from build123d import *

# Parameters (mm, degrees)
SKETCH_1_R          = 2.05
EXTRUDE_1_DEPTH     = 6.5
SKETCH_2_R          = 1.925
CUT_EXTRUDE_1_DEPTH = 46.069390943
SKETCH_4_R          = 3.5
CUT_EXTRUDE_3_DEPTH = 3.7
SKETCH_5_W          = 18.309146901
SKETCH_5_H          = 4.198551417
CUT_EXTRUDE_4_DEPTH = 1.5
CHAMFER_1_SIZE      = 2


with BuildPart() as part:
    # 스케치1 → 보스-돌출1 (new, symmetric)
    with BuildSketch(Plane.XY):
        with BuildLine():
            Line((24, 9.4), (27.233161507, 15))
            Line((27.233161507, 15), (37.358175691, 15))
            Line((37.358175691, 15), (42, 10.358175691))
            Line((42, 10.358175691), (42, 8))
            Line((42, 8), (42, 4.214621821))
            Line((42, 4.214621821), (39.656854249, 2.343145751))
            ThreePointArc((39.656854249, 2.343145751), (37.061467459, 0.60896374), (34, 0))
            Line((34, 0), (0, 0))
            Line((0, 0), (0, 8.847038924))
            Line((0, 8.847038924), (12.898784487, 8.847038924))
            Line((12.898784487, 8.847038924), (13.451745563, 9.4))
            Line((13.451745563, 9.4), (24, 9.4))
        make_face()
        with Locations(Location((34, 10, 0), (0, 0, 180))):
            Circle(SKETCH_1_R, mode=Mode.SUBTRACT)
    extrude(amount=EXTRUDE_1_DEPTH, both=True)

    # 스케치2 → 컷-돌출1 (cut, through all)
    with BuildSketch(Plane(origin=(0, 0, 0), x_dir=(1, 0, 0), z_dir=(0, 1, 0))):
        with Locations(Location((7.95, 0, 0), (0, 0, 90))):
            Circle(SKETCH_2_R)
        with Locations((17.95, 0)):
            Circle(SKETCH_2_R)
    extrude(amount=CUT_EXTRUDE_1_DEPTH, mode=Mode.SUBTRACT)

    # 스케치4 → 컷-돌출3 (cut)
    with BuildSketch(Plane(origin=(0, 9.4, 0), x_dir=(1, 0, 0), z_dir=(0, 1, 0))):
        with Locations(Location((7.95, 0, 0), (0, 0, 270))):
            Circle(SKETCH_4_R)
        with Locations(Location((17.95, 0, 0), (0, 0, 270))):
            Circle(SKETCH_4_R)
    extrude(amount=-CUT_EXTRUDE_3_DEPTH, mode=Mode.SUBTRACT)

    # 스케치5 → 컷-돌출4 (cut, symmetric)
    with BuildSketch(Plane.XY):
        with Locations((31.708331529, 16.176346462)):
            Rectangle(SKETCH_5_W, SKETCH_5_H)
    extrude(amount=CUT_EXTRUDE_4_DEPTH, both=True, mode=Mode.SUBTRACT)

    # 모따기1
    chamfer_1_edges = [part.edges().sort_by_distance(p)[0] for p in [
        (25.616580754, 12.2, -6.5),
        (25.616580754, 12.2, 6.5),
    ]]
    chamfer(chamfer_1_edges, length=CHAMFER_1_SIZE)


solid = part.part
The model under review builds one solid part; all positions refer to its coordinate system, in mm. A direction names the side the tool comes from. Give positions to 0.01 mm unless a question says otherwise; leave off trailing zeros. Order: outer loops, then holes, each group sorted by start corner. A loop starts at its lowest first (then second) coordinate and runs counter-clockwise, first axis right, second up. Notation, with made-up numbers: M -17.75,31 L -6.75,31 A21 cw -6.75,68 Z; hole C 8.25,-24.75 d10. An arc over 180 degrees is marked long. Answer in a Markdown table with one row per item. Add a question column.
1. Add section A-A on z = 0. State the section outline as (x, y) points (3 decimals).
2. Mouldability with a two-part tool opening along X and no side actions: class faces 1 (the flat face through (39.65, 12.71, 0.09)), 2 (the flat face through (17, 0, 3)), 3 (the cylindrical face through (16.42, 2.81, 1.17)) as released by +X, released by -X, zero draft, split by the parting line, or undercut.
3. Add section B-B on y = 7.5. State the section outline as (x, z) points, plus the area to 3 significant figures.
4. Machinability: for faces 4 (the flat face through (32.4, 14.5, -1.5)), 5 (the flat face through (16, 5.7, 2)), 6 (the flat face through (0, 4, 0)), which of the approach directions +Z, -Z, +X, -X, +Y, -Y give a long, thin tool a straight path to every point of the face, cutting with its end or side? Answer none if there is none.
5. For pin 1 Ø6.5 at (x, z) = (7.95, 0) entering from -Y; pin 2 Ø3.5 at (x, y) = (34, 10) entering from +Z; pin 3 Ø4 at (x, z) = (13, 5) entering from +Y; pin 4 Ø2 at (x, z) = (19.5, 1.5) entering from +Y, all flat-tipped, find the tip position at first contact; note any pin that passes through.
6. Add section D-D on y = 10.75. State the section outline as (x, z) points, plus the area to 3 significant figures.
7. To check wall thickness, follow line 1 along X through (y, z) = (7.45, 0); line 2 along Z through (x, y) = (17.95, 1.55) (3 decimals); line 3 along Y through (x, z) = (34, -0.25). State the ranges of each line that lie inside material, in increasing order.
8. Add section C-C on x = 17.95. State the section outline as (y, z) points (3 decimals).
The answers:
| question | item | result |
|---|---|---|
| 1 | outline | M 0,0 L 6.025,0 L 6.025,5.7 L 4.45,5.7 L 4.45,8.847 L 0,8.847 Z; M 9.875,0 L 16.025,0 L 16.025,5.7 L 14.45,5.7 L 14.45,9.4 L 13.452,9.4 L 12.899,8.847 L 11.45,8.847 L 11.45,5.7 L 9.875,5.7 Z; M 19.875,0 L 34,0 A8 ccw 39.657,2.343 L 42,4.215 L 42,10.358 L 38.281,14.077 L 26.7,14.077 L 24,9.4 L 21.45,9.4 L 21.45,5.7 L 19.875,5.7 Z; hole C 34,10 d4.1 |
| 2 | face 1 | released by +X |
| 2 | face 2 | zero draft |
| 2 | face 3 | undercut |
| 3 | outline | M 0,-6.5 L 42,-6.5 L 42,6.5 L 0,6.5 Z; hole C 7.95,0 d7; hole C 17.95,0 d7 |
| 3 | area | 469 mm2 |
| 4 | face 4 | +X, -X, +Y |
| 4 | face 5 | +Y |
| 4 | face 6 | +Z, -Z, -X, +Y, -Y |
| 5 | pin 1 | y = 0 |
| 5 | pin 2 | through |
| 5 | pin 3 | y = 9.4 |
| 5 | pin 4 | y = 5.7 |
| 6 | outline | M 24.78,-4.5 L 27.09,-6.5 L 32.09,-6.5 L 32.09,6.5 L 27.09,6.5 L 24.78,4.5 Z; M 35.91,-6.5 L 41.61,-6.5 L 41.61,6.5 L 35.91,6.5 Z |
| 6 | area | 165 mm2 |
| 7 | line 1 | 0 to 4.45, 11.45 to 14.45, 21.45 to 42 |
| 7 | line 2 | -6.5 to -1.925, 1.925 to 6.5 |
| 7 | line 3 | 0 to 7.95, 12.05 to 14.08 |
| 8 | outline | M 0,-6.5 L 9.4,-6.5 L 9.4,-3.5 L 5.7,-3.5 L 5.7,-1.925 L 0,-1.925 Z; M 0,1.925 L 5.7,1.925 L 5.7,3.5 L 9.4,3.5 L 9.4,6.5 L 0,6.5 Z |
